Could you check a few things on this model? Use its own coordinates, in mm. Face numbers are marked on the shaded views. A direction names the side the tool comes from. Give positions to 0.01 mm unless a question says otherwise; leave off trailing zeros. Loops run counter-clockwise (first coordinate to the right, second up) from the corner with the lowest first, then second, coordinate; pieces in that order, holes last. Notation, with made-up numbers: (19.25, 19) -> (45.25, 19) arc R21 ccw to (45.25, 38) -> close; hole circle Ø4 at (-25.5, 40). An arc over 180 degrees is marked (long way). Write item = value, one per line. Start each with the question number.
1) I want a section at A-A (x = 12.5). List the corners of the cut face in (y, z) for me.
2) I want a section at B-B (y = -16). Count the separate pieces of the cut face and the enclosed holes in it, and give its area (3 significant figures).
3) I need wall thicknesses on probe 1 along Y at (x, z) = (-7, 5.25); probe 2 along Y at (x, z) = (5, 3.75); probe 3 along X at (y, z) = (-25.5, 4.5). Which ranges of each line are inside material? Lowest first, please. Write a range as from..to.
4) On a 3-axis mill with a long thin cutter (end or side, diameter ignored), from which of +Z, -Z, +X, -X, +Y, -Y can I reach the whole of each face in a straight line? I mean the marked faces 1, 2, 3 and 4. Say none if no direction works.
5) If we mould it in two halves opening along Y, with no side actions, what happens to the marked faces 5, 6, 7 and 8? For each: +Y half, -Y half, draft (parallel to the pull), parting line (faces both ways), or undercut.
6) I'm going to push flat-ended pins straight in: pin 1 Ø1.5 at (y, z) = (-1.5, 5.5) entering from -X; pin 2 Ø1.5 at (y, z) = (3, 11.5) entering from -X; pin 3 Ø1.5 at (x, z) = (10, 5) entering from +Y. Where does each tip first touch, or does it pass through?
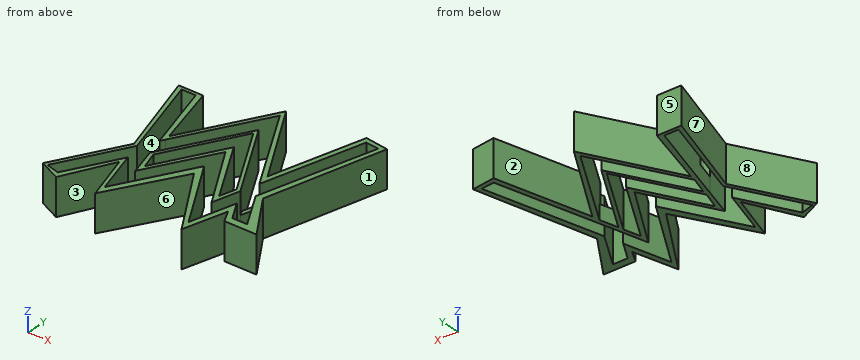
from build123d import *

# Parameters (mm, degrees)
F1_DEPTH = 12.7
F2_DEPTH = 5.08


with BuildPart() as f1:
    # F0 (on Top) → F1 (new body)
    with BuildSketch(Plane.XY):
        Polygon((-20.5210409951, -7.9736062909), (-33.5891470313, -30.8521799743), (-26.4399256557, -34.2453196645), (-17.9045014083, -17.60189794), (-13.0402278155, -34.2453196645), (1.5525938943, -9.8924823105), (16.5106914937, -34.2453196645), (20.7147076726, -19.4195080549), (22.9475684464, -23.8377209753), (33.9693464339, -23.8377209753), (23.9674728364, -8.3760125563), (34.5444940031, 31.9929458201), (26.6998670995, 33.0506488681), (17.9738253355, 1.2314473279), (1.3111314686, 30.3455736883), (-15.5200697482, 0.8788800333), (-21.1611483246, 22.8261984885), (-29.5346230268, 22.8261984885), align=None)
        Polygon((-27.5588259101, -32.1146920323), (-32.0720225573, -30.8284889907), (-19.2177128047, -8.3242123947), (-27.6659652591, 21.6798372567), (-22.7880645543, 21.6798372567), (-16.0654503852, -2.5953715667), (-15.1892008377, -1.078940688), (1.3588338625, 27.5589637458), (17.5643963544, -1.3110835766), (18.5902547091, -3.1386399642), (28.0608907342, 31.214652583), (32.5249694288, 30.7627916336), (21.6690897942, -8.6306408048), (28.7532173097, -21.3059335947), (23.7063355744, -21.3059335947), (19.992057234, -14.7041222081), (15.7005265355, -30.1691573113), (1.3588338625, -5.2477028221), (-13.042463921, -30.1347691566), (-17.4419488758, -14.6160917357), (-17.4973364919, -14.3933231011), align=None, mode=Mode.SUBTRACT)
    extrude(amount=F1_DEPTH)



with BuildPart() as f1b:
    # F0 (on Top) → F1, piece 2 (new body)
    with BuildSketch(Plane.XY):
        Polygon((-13.348367419, -7.1639683075), (-14.3312010466, -8.8577069897), (-14.3479155377, -8.8865114376), (-11.6898040163, -18.593637318), (1.3742336305, 3.9824927226), (14.3406316638, -18.4643995017), (16.8852303177, -9.2208087444), (15.8592973644, -7.3935184654), (1.4307427919, 18.3051954955), align=None)
        Polygon((-11.1567043809, -15.1034206777), (-13.0402278155, -9.0519273654), (1.3387252224, 16.1215702828), (15.4962225923, -9.0943634049), (13.9230203858, -14.6423914203), (1.6215687562, 7.2677372167), align=None, mode=Mode.SUBTRACT)
    extrude(amount=F1_DEPTH)


with BuildPart() as f1_1:
    add(f1.part)

    add(f1b.part)  # F2 merges F1b
    # F0 (on Top) → F2 (join)
    with BuildSketch(Plane.XY):
        Polygon((-15.1892008377, -1.078940688), (-16.0654503852, -2.5953715667), (-14.3312010466, -8.8577069897), (-13.348367419, -7.1639683075), align=None)
        Polygon((18.5902547091, -3.1386399642), (17.5643963544, -1.3110835766), (15.8592973644, -7.3935184654), (16.8852303177, -9.2208087444), align=None)
    extrude(amount=F2_DEPTH)


solid = f1_1.part
Answer list:
q1.outline = (-27.72, 0) -> (-24.61, 0) -> (-24.61, 12.7) -> (-27.72, 12.7) -> close; (-15.28, 0) -> (-12.11, 0) -> (-12.11, 12.7) -> (-15.28, 12.7) -> close; (-3.76, 0) -> (-1.41, 0) -> (-1.41, 12.7) -> (-3.76, 12.7) -> close; (7.71, 0) -> (10.8, 0) -> (10.8, 12.7) -> (7.71, 12.7) -> close
q2.separate_pieces = 8
q2.enclosed_holes = 0
q2.area = 208 mm^2
q3.probe_1 = -24.17..-19.69, -10.49..-7.83, 1.52..3.78, 13.09..15.8
q3.probe_2 = -15.51..-11.57, -2.29..1.25, 9.6..11.95, 21.07..23.9
q3.probe_3 = -30.53..-29.03, -23.8..-21.95, -15.6..-14.36, -10.36..-7.8, 11.14..13.01, 17..18.99
q4.face_1 = +Z, -Z, +X
q4.face_2 = +Z, -Z, +Y
q4.face_3 = +Z, -Z, -Y
q4.face_4 = +Z, -Z
q5.face_5 = +Y half
q5.face_6 = -Y half
q5.face_7 = undercut
q5.face_8 = undercut
q6.pin_1 = -22.64
q6.pin_2 = -23.95
q6.pin_3 = 16.47
